Verification items for the finished model (mm, model axes). A direction names the side the tool comes from. Round coordinates to 2 decimals unless told otherwise and drop trailing zeros. Order: outer loops, then holes, each group sorted by start corner. A loop starts at its lowest first (then second) coordinate and runs counter-clockwise, first axis right, second up. Notation, with made-up numbers: (38, 25) -> (97, 25) arc R25 cw to (97, 50) -> close; hole circle Ø9 at (51.5, -10). An arc over 180 degrees is marked (long way). Return JSON: item names as keys, results as strings. Group by question number.
Item 1: Sectioned sample at C-C on x = -12. Record the cut outline in (y, z), plus the area to 3 significant figures.
Item 2: Scan lines: probe 1 along Z at (x, y) = (12, 3.75); probe 2 along X at (y, z) = (2.05, 0); probe 3 along Z at (x, y) = (-12, 9.25). Record each from-to range of solid material in increasing order. Write a range as from..to.
Item 3: Access from +Z, -Z, +X, -X, +Y, -Y to the whole of each face (thin tool, end or side, straight path). Record for faces 4 (the flat face through (-15, 0.75, 0)), 5 (the flat face through (-12, 6, 3)).
Item 4: Sectioned sample at D-D on y = 10. Record the cut outline in (x, z).
Item 5: Sectioned sample at A-A on z = 0. Record the cut outline in (x, y), plus the area to 3 significant figures.
Item 6: Sectioned sample at B-B on y = 3.25. Record the cut outline in (x, z), plus the area to 3 significant figures.
Item 7: Draft check along Z on faces 1 (the flat face through (0, 9, 6)), 2 (the cylindrical face through (0, 8, 0)), 3 (the flat face through (12, 6, 3)). Enter one of: pulls with the +Z half, pulls with the -Z half, needs draft (parallel to the pull), parting line crosses it, or undercut.
Item 8: Depth check by flat-ended pin: pin 1 Ø3 at (y, z) = (8, -1.5) entering from +X; pin 2 Ø5 at (x, z) = (12, 0) entering from +Y; pin 3 Ø2 at (y, z) = (6, 0) entering from -X; pin 4 Ø7 at (x, z) = (-12, 0) entering from +Y. Enter the tip coordinate at first touch or a pass-through.
```python
from build123d import *

# Parameters (mm, degrees)
EXTRUDE_1_DEPTH     = 6
SKETCH_2_R          = 2.75
CUT_EXTRUDE_1_DEPTH = 25.944939367
CUT_EXTRUDE_START   = 6
SKETCH_3_R          = 4.5
CUT_EXTRUDE_2_DEPTH = 20.454616638


with BuildPart() as part:
    # 草图1 → 凸台-拉伸1 (new, symmetric)
    with BuildSketch(Plane.XY):
        with BuildLine():
            Line((-17.483921185, 0.75), (-7.964766161, 0.75))
            ThreePointArc((-7.964766161, 0.75), (0, 8), (7.964766161, 0.75))
            Line((7.964766161, 0.75), (17.483921185, 0.75))
            ThreePointArc((17.483921185, 0.75), (0, 17.5), (-17.483921185, 0.75))
        make_face()
    extrude(amount=EXTRUDE_1_DEPTH, both=True)

    # 草图2 → 切除-拉伸1 (cut, through all)
    with BuildSketch(Plane.XZ.offset(-0.75)):
        with Locations(Location((-12, 0, 0), (0, 0, 270))):
            Circle(SKETCH_2_R)
    cut_extrude_1 = extrude(amount=-CUT_EXTRUDE_1_DEPTH, mode=Mode.SUBTRACT)

    # 草图3 → 切除-拉伸2 (cut, through all)
    with BuildSketch(Plane(origin=(0, 0, 0), x_dir=(1, 0, 0), z_dir=(0, 1, 0)).offset(CUT_EXTRUDE_START)):
        with Locations((-12, 0)):
            Circle(SKETCH_3_R)
    cut_extrude_2 = extrude(amount=CUT_EXTRUDE_2_DEPTH, mode=Mode.SUBTRACT)

    # 镜向1: 切除-拉伸1, 切除-拉伸2 across plane
    add(cut_extrude_1.mirror(Plane(origin=(0, 0, 0), x_dir=(0, 0, 1), z_dir=(1, 0, 0))), mode=Mode.SUBTRACT)
    add(cut_extrude_2.mirror(Plane(origin=(0, 0, 0), x_dir=(0, 0, 1), z_dir=(1, 0, 0))), mode=Mode.SUBTRACT)


solid = part.part
```
Recorded:
{
 "1": {"outline": "(0.75, -6) -> (12.74, -6) -> (12.74, -4.5) -> (6, -4.5) -> (6, -2.75) -> (0.75, -2.75) -> close; (0.75, 2.75) -> (6, 2.75) -> (6, 4.5) -> (12.74, 4.5) -> (12.74, 6) -> (0.75, 6) -> close", "area": "54.3 mm²"},
 "2": {"probe 1": "-6..-2.75, 2.75..6", "probe 2": "-17.38..-14.75, -9.25..-7.73, 7.73..9.25, 14.75..17.38", "probe 3": "-6..-4.5, 4.5..6"},
 "3": {"face 4": "+Z, -Z, +X, -X, -Y", "face 5": "+Y"},
 "4": {"outline": "(-14.36, -6) -> (14.36, -6) -> (14.36, -3.83) arc R4.5 cw (long way) to (14.36, 3.83) -> (14.36, 6) -> (-14.36, 6) -> (-14.36, 3.83) arc R4.5 cw (long way) to (-14.36, -3.83) -> close"},
 "5": {"outline": "(-17.48, 0.75) -> (-14.75, 0.75) -> (-14.75, 6) -> (-16.44, 6) arc R17.5 ccw to start; (-9.25, 0.75) -> (-7.96, 0.75) arc R8 cw to (7.96, 0.75) -> (9.25, 0.75) -> (9.25, 6) -> (7.5, 6) -> (7.5, 15.81) arc R17.5 ccw to (-7.5, 15.81) -> (-7.5, 6) -> (-9.25, 6) -> close; (14.75, 0.75) -> (17.48, 0.75) arc R17.5 ccw to (16.44, 6) -> (14.75, 6) -> close", "area": "197 mm²"},
 "6": {"outline": "(-17.2, -6) -> (-7.31, -6) -> (-7.31, 6) -> (-17.2, 6) -> close; (7.31, -6) -> (17.2, -6) -> (17.2, 6) -> (7.31, 6) -> close; hole circle Ø5.5 at (-12, 0); hole circle Ø5.5 at (12, 0)", "area": "190 mm²"},
 "7": {"face 1": "pulls with the +Z half", "face 2": "needs draft", "face 3": "undercut"},
 "8": {"pin 1": "x = 16.25", "pin 2": "through", "pin 3": "x = -16.77", "pin 4": "y = 6"}
}
